from build123d import *

# Parameters (mm, degrees)
SKETCH1_W               = 55
SKETCH1_H               = 80
BOSS_EXTRUDE1_DEPTH     = 10
SKETCH6_R               = 1.65
CUT_EXTRUDE2_DEPTH      = 55
LPATTERN1_COUNT         = 3
LPATTERN1_PITCH         = 25
MIRROR3_COPY_1_SKETCH_R = 1.65
MIRROR3_COPY_1_DEPTH    = 55
MIRROR3_COPY_2_SKETCH_R = 1.65
MIRROR3_COPY_2_DEPTH    = 55
SKETCH8_W               = 8
SKETCH8_H               = 55
BOSS_EXTRUDE3_DEPTH     = 65
FILLET3_R               = 5
SKETCH9_R               = 1.6
SKETCH9_R_2             = 11.5
CUT_EXTRUDE3_DEPTH      = 32.5
SKETCH10_R              = 3
CUT_EXTRUDE4_DEPTH      = 3
CUT_EXTRUDE5_START      = -5
SKETCH11_R              = 3
CUT_EXTRUDE5_DEPTH      = 71
LPATTERN2_COUNT         = 3
LPATTERN2_PITCH         = 25
MIRROR4_START           = -5
MIRROR4_COPY_1_SKETCH_R = 3
MIRROR4_COPY_1_DEPTH    = 71
MIRROR4_COPY_2_SKETCH_R = 3
MIRROR4_COPY_2_DEPTH    = 71
CUT_EXTRUDE6_DEPTH      = 10
SKETCH13_R              = 4.15
BOSS_EXTRUDE4_DEPTH     = 23.5


with BuildPart() as part:
    # Sketch1 → Boss-Extrude1 (new body)
    with BuildSketch(Plane(origin=(0, 0, 0), x_dir=(1, 0, 0), z_dir=(0, 1, 0))):
        Rectangle(SKETCH1_W, SKETCH1_H)
    extrude(amount=BOSS_EXTRUDE1_DEPTH)

    # Sketch6 → Cut-Extrude2 (cut)
    with BuildSketch(Plane(origin=(0, 10, 0), x_dir=(1, 0, 0), z_dir=(0, 1, 0))):
        with Locations((-12.5, -25)):
            Circle(SKETCH6_R)
    cut_extrude2 = extrude(amount=-CUT_EXTRUDE2_DEPTH, mode=Mode.SUBTRACT)

    # LPattern1: Cut-Extrude2 ×3
    with Locations(*[(0, 0, -i * LPATTERN1_PITCH) for i in range(1, LPATTERN1_COUNT)]):
        add(cut_extrude2, mode=Mode.SUBTRACT)

    # Mirror3: Cut-Extrude2 across plane
    add(cut_extrude2.mirror(Plane(origin=(0, 0, 0), x_dir=(0, 0, 1), z_dir=(1, 0, 0))), mode=Mode.SUBTRACT)

    # Mirror3 copy 1 sketch → Mirror3 copy 1 (cut)
    with BuildSketch(Plane(origin=(0, 10, -25), x_dir=(-1, 0, 0), z_dir=(0, 1, 0))):
        with Locations((-12.5, 25)):
            Circle(MIRROR3_COPY_1_SKETCH_R)
    extrude(amount=-MIRROR3_COPY_1_DEPTH, mode=Mode.SUBTRACT)

    # Mirror3 copy 2 sketch → Mirror3 copy 2 (cut)
    with BuildSketch(Plane(origin=(0, 10, -50), x_dir=(-1, 0, 0), z_dir=(0, 1, 0))):
        with Locations((-12.5, 25)):
            Circle(MIRROR3_COPY_2_SKETCH_R)
    extrude(amount=-MIRROR3_COPY_2_DEPTH, mode=Mode.SUBTRACT)

    # Sketch8 → Boss-Extrude3 (add)
    with BuildSketch(Plane(origin=(0, 10, 0), x_dir=(1, 0, 0), z_dir=(0, 1, 0))):
        Rectangle(SKETCH8_W, SKETCH8_H)
    extrude(amount=BOSS_EXTRUDE3_DEPTH)

    # Fillet3
    fillet3_edges = [part.edges().sort_by_distance(p)[0] for p in [
        (4, 10, 0),
        (0, 10, -27.5),
        (-4, 10, 0),
        (0, 10, 27.5),
        (0, 75, -27.5),
        (0, 75, 27.5),
        (-27.5, 5, -40),
        (27.5, 5, -40),
    ]]
    fillet(fillet3_edges, radius=FILLET3_R)

    # Sketch9 → Cut-Extrude3 (cut, through all)
    with BuildSketch(Plane.ZY.offset(4)):
        with Locations((-15.5, 65.5)):
            Circle(SKETCH9_R)
        with Locations((15.5, 65.5)):
            Circle(SKETCH9_R)
        with Locations((-15.5, 34.5)):
            Circle(SKETCH9_R)
        with Locations((15.5, 34.5)):
            Circle(SKETCH9_R)
        with Locations((0, 50)):
            Circle(SKETCH9_R_2)
    extrude(amount=-CUT_EXTRUDE3_DEPTH, mode=Mode.SUBTRACT)

    # Sketch10 → Cut-Extrude4 (cut)
    with BuildSketch(Plane(origin=(4, 0, 0), x_dir=(0, 0, -1), z_dir=(1, 0, 0))):
        with Locations((-15.5, 65.5)):
            Circle(SKETCH10_R)
        with Locations((15.5, 65.5)):
            Circle(SKETCH10_R)
        with Locations((15.5, 34.5)):
            Circle(SKETCH10_R)
        with Locations((-15.5, 34.5)):
            Circle(SKETCH10_R)
    extrude(amount=-CUT_EXTRUDE4_DEPTH, mode=Mode.SUBTRACT)

    # Sketch11 → Cut-Extrude5 (cut)
    with BuildSketch(Plane(origin=(0, 10, 0), x_dir=(1, 0, 0), z_dir=(0, 1, 0)).offset(CUT_EXTRUDE5_START)):
        with Locations((-12.5, -25)):
            Circle(SKETCH11_R)
    cut_extrude5 = extrude(amount=CUT_EXTRUDE5_DEPTH, mode=Mode.SUBTRACT)

    # LPattern2: Cut-Extrude5 ×3
    with Locations(*[(0, 0, -i * LPATTERN2_PITCH) for i in range(1, LPATTERN2_COUNT)]):
        add(cut_extrude5, mode=Mode.SUBTRACT)

    # Mirror4: Cut-Extrude5 across plane
    add(cut_extrude5.mirror(Plane(origin=(0, 0, 0), x_dir=(0, 0, 1), z_dir=(1, 0, 0))), mode=Mode.SUBTRACT)

    # Mirror4 copy 1 sketch → Mirror4 copy 1 (cut)
    with BuildSketch(Plane(origin=(0, 10, -25), x_dir=(-1, 0, 0), z_dir=(0, 1, 0)).offset(MIRROR4_START)):
        with Locations((-12.5, 25)):
            Circle(MIRROR4_COPY_1_SKETCH_R)
    extrude(amount=MIRROR4_COPY_1_DEPTH, mode=Mode.SUBTRACT)

    # Mirror4 copy 2 sketch → Mirror4 copy 2 (cut)
    with BuildSketch(Plane(origin=(0, 10, -50), x_dir=(-1, 0, 0), z_dir=(0, 1, 0)).offset(MIRROR4_START)):
        with Locations((-12.5, 25)):
            Circle(MIRROR4_COPY_2_SKETCH_R)
    extrude(amount=MIRROR4_COPY_2_DEPTH, mode=Mode.SUBTRACT)

    # Sketch12 → Cut-Extrude6 (cut)
    with BuildSketch(Plane(origin=(0, 10, 0), x_dir=(1, 0, 0), z_dir=(0, 1, 0))):
        Polygon((12.5, -37), (-38.055736231, -37), (-38.055736231, -44.287300659), (40.369344369, -44.287300659), (40.369344369, -37), align=None)
    extrude(amount=-CUT_EXTRUDE6_DEPTH, mode=Mode.SUBTRACT)

    # Sketch13 → Boss-Extrude4 (add)
    with BuildSketch(Plane(origin=(4, 0, 0), x_dir=(0, 0, -1), z_dir=(1, 0, 0))):
        with BuildLine():
            Line((-7.35, 25), (-7.35, 10))
            Line((-7.35, 10), (-7.35, 0))
            Line((-7.35, 0), (7.35, 0))
            Line((7.35, 0), (7.35, 10))
            Line((7.35, 10), (7.35, 25))
            ThreePointArc((7.35, 25), (0, 32.35), (-7.35, 25))
        make_face()
        with Locations((0, 25)):
            Circle(SKETCH13_R, mode=Mode.SUBTRACT)
    extrude(amount=BOSS_EXTRUDE4_DEPTH)


solid = part.part
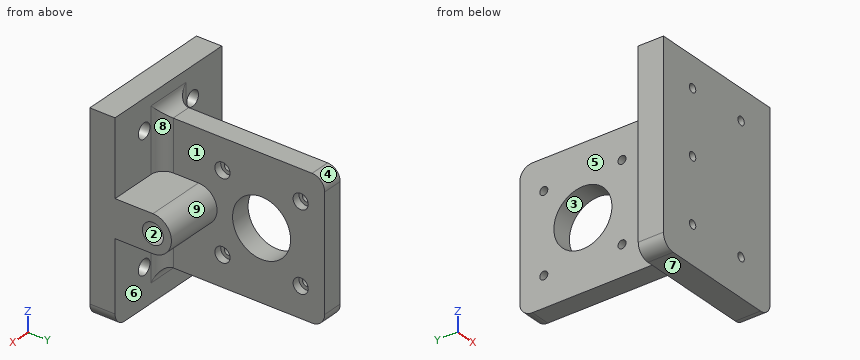
Input: part model. Units: mm. Frame: model coordinates. Face numbers are marked on the shaded views. A direction names the side the tool comes from. Give positions to 0.01 mm unless a question says otherwise; leave off trailing zeros. Write each loop counter-clockwise with the first axis right and the second up, starting at its lowest first coordinate (ties: lowest second). Pieces come first, ordered by that corner, then holes.
Q1. Section C-C, the plane x = 17. Output: boundary loops of the cut face in (y, z).
Q2. Section A-A, the plane y = 50. Output: boundary loops of the cut face in (x, z).
Q3. Pull-direction query (Z, two-part tool) for the marked faces 1, 2, 3 and 4; classes: pulls with the +Z half, pulls with the -Z half, needs draft (parallel to the pull), parting line crosses it, or undercut.
Q4. Set-up query: the marked faces 5, 6, 7, 8 and 9. Return all of +Z, -Z, +X, -X, +Y, -Y with unobstructed straight access to the full face (end or side cutting, diameter ignored); none if empty.
Q5. Section B-B, the plane z = -15.5. Output: boundary loops of the cut face in (x, y).
Q6. Section D-D, the plane y = 34.5. Output: boundary loops of the cut face in (x, z).
Q7. First-contact query: P1, Ø6.5, axis at x = 1.5, y = 52.5, coming from the -Z side; P2, Ø5, axis at y = 34.5, z = 15.5, coming from the +X side; P3, Ø6, axis at y = 16.5, z = 13, coming from the +X side. Flat tips, straight axial feed; report the tip coordinate or a pass-through.
Q8. Material intervals for probe 1 along Z at (x, y) = (-1.5, 65.5); probe 2 along Y at (x, z) = (-25, 27); probe 3 along Z at (x, y) = (-12, 6), sorted ascending.
Filled in:
1. outline: (0, -40) - (10, -40) - (10, -7.35) - (25, -7.35) arc R7.35 ccw to (25, 7.35) - (10, 7.35) - (10, 37) - (0, 37) - close; hole circle Ø8.3 at (25, 0)
2. outline: (-4, -27.5) - (4, -27.5) - (4, -11.5) - (-4, -11.5) - close; (-4, 11.5) - (4, 11.5) - (4, 27.5) - (-4, 27.5) - close
3. face 1: needs draft
3. face 2: undercut
3. face 3: undercut
3. face 4: pulls with the +Z half
4. face 5: +Z, -Z, -X, +Y
4. face 6: +Y
4. face 7: -Z, +X, -X, +Y, -Y
4. face 8: +Z, +X, +Y
4. face 9: +X, +Y
5. outline: (-27.5, 0) - (27.5, 0) - (27.5, 10) - (9, 10) arc R5 cw to (4, 15) - (4, 31.5) - (1, 31.5) - (1, 32.9) - (-4, 32.9) - (-4, 15) arc R5 cw to (-9, 10) - (-27.5, 10) - close; (-4, 36.1) - (1, 36.1) - (1, 37.5) - (4, 37.5) - (4, 62.5) - (1, 62.5) - (1, 63.9) - (-4, 63.9) - close; (-4, 67.1) - (1, 67.1) - (1, 68.5) - (4, 68.5) - (4, 75) - (-4, 75) - close
6. outline: (-4, -27.5) - (4, -27.5) - (4, -18.5) - (1, -18.5) - (1, -17.1) - (-4, -17.1) - close; (-4, -13.9) - (1, -13.9) - (1, -12.5) - (4, -12.5) - (4, 12.5) - (1, 12.5) - (1, 13.9) - (-4, 13.9) - close; (-4, 17.1) - (1, 17.1) - (1, 18.5) - (4, 18.5) - (4, 27.5) - (-4, 27.5) - close
7. P1: stops at z = -27.5
7. P2: stops at x = 1
7. P3: stops at x = 4.23
8. probe 1: z = -27.5 to -17.1, -13.9 to 13.9, 17.1 to 27.5
8. probe 2: y = 0 to 10
8. probe 3: z = -40 to -27.96, -22.04 to -2.96, 2.96 to 22.04, 27.96 to 37
